from build123d import *

# Parameters (mm, degrees)
EXTRUDE1_DEPTH     = 12.7
SKETCH2_R          = 17.78
CUT_EXTRUDE1_DEPTH = 242.3


with BuildPart() as part:
    # Sketch1 → Extrude1 (new body)
    with BuildSketch(Plane.XY):
        Polygon((-76.2, 215.9), (-53.975, 215.9), (-53.975, 228.6), (-34.925, 228.6), (-34.925, 215.9), (34.925, 215.9), (34.925, 228.6), (53.975, 228.6), (53.975, 215.9), (76.2, 215.9), (76.2, 142.24), (-76.2, 142.24), align=None)
    extrude(amount=-EXTRUDE1_DEPTH)

    # Sketch2 → Cut-Extrude1 (cut, through all)
    with BuildSketch(Plane.XY):
        with Locations((0, 142.24)):
            Circle(SKETCH2_R)
    extrude(amount=-CUT_EXTRUDE1_DEPTH, mode=Mode.SUBTRACT)


solid = part.part
Work out the finished part from the listing and answer in its coordinate system (mm). A direction names the side the tool comes from. Give positions to 0.01 mm unless a question says otherwise; leave off trailing zeros. Loops run counter-clockwise (first coordinate to the right, second up) from the corner with the lowest first, then second, coordinate; pieces in that order, holes last. Notation, with made-up numbers: (-21.5, 58) -> (-10.5, 58) arc R36 ccw to (-10.5, 93) -> close; hole circle Ø6 at (-27.75, -12). An arc over 180 degrees is marked (long way). Use a Markdown table: item, result. Add a question column.
1) The part is cut by section C-C, the plane x = 0. Determine the outline of the cut face in (y, z).
2) The part is cut by section B-B, the plane x = -63. Determine the outline of the cut face in (y, z), plus the area to 3 significant figures.
3) For a pull along X with two mould halves and no side action, classify faces 1 (the flat face through (-47, 142.24, -6)), 2 (the flat face through (76.2, 180, -6)), 3 (the flat face through (34.925, 222, -6)) as +X half, -X half, draft (parallel to the pull), parting line (faces both ways), or undercut.
4) The part is cut by section A-A, the plane z = -6.75. Determine the outline of the cut face in (x, y) (3 decimals).
5) Consider line 1 along Y through (x, z) = (61.5, -1.75); line 2 along Y through (x, z) = (1, -9.5); line 3 along X through (y, z) = (155.5, -3.25). Determine where each line is inside the solid, lowest interval first.
6) Each of these flat-tipped pins is pushed along its axis until it touches: P1, Ø4, axis at x = 54, z = -2, coming from the +Y side; P2, Ø4, axis at x = -7.5, z = -7.5, coming from the +Y side; P3, Ø6.5, axis at y = 221, z = -8.5, coming from the +X side (3 decimals); P4, Ø6.5, axis at y = 221.5, z = -9.5, coming from the -X side (3 decimals). Where does it stop, or does it pass through?
7) Which of the six approach directions +Z, -Z, +X, -X, +Y, -Y give full straight-line access (tool end or side, diameter ignored) to faces 4 (the flat face through (65, 215.9, -6)), 5 (the flat face through (-34.925, 222, -6)), 6 (the flat face through (-53.975, 222, -6))?
Reported:
| question | item | result |
|---|---|---|
| 1 | outline | (160.02, -12.7) -> (215.9, -12.7) -> (215.9, 0) -> (160.02, 0) -> close |
| 2 | outline | (142.24, -12.7) -> (215.9, -12.7) -> (215.9, 0) -> (142.24, 0) -> close |
| 2 | area | 935 mm^2 |
| 3 | face 1 | draft |
| 3 | face 2 | +X half |
| 3 | face 3 | undercut |
| 4 | outline | (-76.2, 142.24) -> (-17.78, 142.24) arc R17.78 cw to (17.78, 142.24) -> (76.2, 142.24) -> (76.2, 215.9) -> (53.975, 215.9) -> (53.975, 228.6) -> (34.925, 228.6) -> (34.925, 215.9) -> (-34.925, 215.9) -> (-34.925, 228.6) -> (-53.975, 228.6) -> (-53.975, 215.9) -> (-76.2, 215.9) -> close |
| 5 | line 1 | y = 142.24 to 215.9 |
| 5 | line 2 | y = 159.99 to 215.9 |
| 5 | line 3 | x = -76.2 to -11.84, 11.84 to 76.2 |
| 6 | P1 | stops at y = 228.6 |
| 6 | P2 | stops at y = 215.9 |
| 6 | P3 | stops at x = 53.975 |
| 6 | P4 | stops at x = -53.975 |
| 7 | face 4 | +Z, -Z, +X, +Y |
| 7 | face 5 | +Z, -Z, +Y |
| 7 | face 6 | +Z, -Z, -X, +Y |
